Source: CAD feature listing. Evaluate the final solid. Frame: model axes, mm. Give positions to 0.01 mm unless a question says otherwise; leave off trailing zeros. Write each loop counter-clockwise with the first axis right and the second up, starting at its lowest first coordinate (ties: lowest second). Pieces come first, ordered by that corner, then holes. Notation, with made-up numbers: (-36.5, 14.25) -> (-17.5, 14.25) arc R5 ccw to (-17.5, 21.25) -> close; hole circle Ø3 at (18, -29.75). An arc over 180 degrees is marked (long way). Use one line per item in the form item = value. Start each with the question number.
(1) Cut plane A-A, the plane z = -390.5. Output: boundary loops of the cut face in (x, y) (3 decimals), and give its area (3 significant figures).
(2) Material intervals for line 1 along Z through (x, y) = (0.5, 4.25); line 2 along Z through (x, y) = (-2.25, -4.25); line 3 along Y through (x, z) = (-0.5, -454.5), sorted ascending. Write a range as from..to.
(3) First-contact query: P1, Ø6, axis at y = -1, z = -498.5, coming from the +X side; P2, Ø6, axis at x = -4.5, y = 4.5, coming from the -Z side; P3, Ø3, axis at x = 3, z = -450.5, coming from the -Y side. Flat tips, straight axial feed; report the tip coordinate or a pass-through.
from build123d import *

# Parameters (mm, degrees)
EXTRUDE1_DEPTH          = 7.9375
SKETCH13_R              = 6.35
EXTRUDE3_DEPTH          = 1.5875
SKETCH2_OUTSIDE_W       = 63.61
SKETCH2_OUTSIDE_H       = 63.61
SKETCH2_OUTSIDE_R       = 4.7625
CUT_EXTRUDE1_DEPTH      = 12.985362166
CUT_EXTRUDE1_DRAFT      = -60
SKETCH14_R              = 1.905
BOSS_EXTRUDE1_DEPTH     = 4.826
MIRROR1_COPY_1_SKETCH_W = 63.61
MIRROR1_COPY_1_SKETCH_H = 63.61
MIRROR1_COPY_1_SKETCH_R = 4.7625
MIRROR1_COPY_1_DEPTH    = 12.985362166
MIRROR1_COPY_1_DRAFT    = -60
SKETCH15_R              = 1.905
BOSS_EXTRUDE2_DEPTH     = 225.298
MIRROR2_COPY_1_SKETCH_W = 63.61
MIRROR2_COPY_1_SKETCH_H = 63.61
MIRROR2_COPY_1_SKETCH_R = 4.7625
MIRROR2_COPY_1_DEPTH    = 12.985362166
MIRROR2_COPY_1_DRAFT    = -60
MIRROR2_COPY_2_DEPTH    = 7.9375
MIRROR2_COPY_3_SKETCH_R = 6.35
MIRROR2_COPY_3_DEPTH    = 1.5875
MIRROR2_COPY_4_SKETCH_R = 1.905
MIRROR2_COPY_4_DEPTH    = 4.826
MIRROR2_COPY_5_SKETCH_W = 63.61
MIRROR2_COPY_5_SKETCH_H = 63.61
MIRROR2_COPY_5_SKETCH_R = 4.7625
MIRROR2_COPY_5_DEPTH    = 12.985362166
MIRROR2_COPY_5_DRAFT    = -60
SKETCH16_R              = 1.905
BOSS_EXTRUDE3_DEPTH     = 3.175
SKETCH4_R               = 1.905
BOSS_EXTRUDE4_DEPTH     = 3.175


with BuildPart() as part:
    # Sketch1 → Extrude1 (new body)
    with BuildSketch(Plane.XY):
        Polygon((0, 5.499261314), (-4.7625, 2.749630657), (-4.7625, -2.749630657), (0, -5.499261314), (4.7625, -2.749630657), (4.7625, 2.749630657), align=None)
    extrude1 = extrude(amount=-EXTRUDE1_DEPTH)

    # Sketch13 → Extrude3 (add)
    with BuildSketch(Plane(origin=(0, 0, -7.9375), x_dir=(-1, 0, 0), z_dir=(0, 0, -1))):
        Circle(SKETCH13_R)
    extrude3 = extrude(amount=-EXTRUDE3_DEPTH)


with BuildPart() as cut_extrude1_tool:
    # Sketch2 outside → Cut-Extrude1 (with draft: the straight prism first)
    with BuildSketch(Plane.XY):
        Rectangle(SKETCH2_OUTSIDE_W, SKETCH2_OUTSIDE_H)
        Circle(SKETCH2_OUTSIDE_R, mode=Mode.SUBTRACT)
    extrude(amount=-CUT_EXTRUDE1_DEPTH)
    # Cut-Extrude1: the draft: its side faces are tilted about the plane it starts from
    cut_extrude1_sides = [cut_extrude1_tool.faces().sort_by_distance(p)[0] for p in [
        (0, -31.805, -6.492681083),
        (31.805, 0, -6.492681083),
        (0, 31.805, -6.492681083),
        (-31.805, 0, -6.492681083),
        (-4.7625, 0, -6.492681083),
    ]]
    draft(cut_extrude1_sides, Plane.XY, CUT_EXTRUDE1_DRAFT)


with BuildPart() as part_1:
    add(part.part)

    # Cut-Extrude1: cut by cut_extrude1_tool
    add(cut_extrude1_tool.part, mode=Mode.SUBTRACT)

    # Sketch14 → Boss-Extrude1 (add)
    with BuildSketch(Plane(origin=(0, 0, -7.9375), x_dir=(-1, 0, 0), z_dir=(0, 0, -1))):
        Circle(SKETCH14_R)
    boss_extrude1 = extrude(amount=BOSS_EXTRUDE1_DEPTH)

    # Mirror1: Extrude1, Extrude3, Boss-Extrude1 across plane
    add(extrude1.mirror(Plane(origin=(0, 0, -12.7635), x_dir=(1, 0, 0), z_dir=(0, 0, -1))))
    add(extrude3.mirror(Plane(origin=(0, 0, -12.7635), x_dir=(1, 0, 0), z_dir=(0, 0, -1))))
    add(boss_extrude1.mirror(Plane(origin=(0, 0, -12.7635), x_dir=(1, 0, 0), z_dir=(0, 0, -1))))


with BuildPart() as mirror1_copy_1_tool:
    # Mirror1 copy 1 sketch → Mirror1 copy 1 (with draft: the straight prism first)
    with BuildSketch(Plane(origin=(0, 0, -25.527), x_dir=(1, 0, 0), z_dir=(0, 0, -1))):
        Rectangle(MIRROR1_COPY_1_SKETCH_W, MIRROR1_COPY_1_SKETCH_H)
        Circle(MIRROR1_COPY_1_SKETCH_R, mode=Mode.SUBTRACT)
    extrude(amount=-MIRROR1_COPY_1_DEPTH)
    # Mirror1 copy 1: the draft: its side faces are tilted about the plane it starts from
    mirror1_copy_1_sides = [mirror1_copy_1_tool.faces().sort_by_distance(p)[0] for p in [
        (0, -31.805, -19.034318917),
        (31.805, 0, -19.034318917),
        (0, 31.805, -19.034318917),
        (-31.805, 0, -19.034318917),
        (-4.7625, 0, -19.034318917),
    ]]
    draft(mirror1_copy_1_sides, Plane(origin=(0, 0, -25.527), x_dir=(1, 0, 0), z_dir=(0, 0, -1)), MIRROR1_COPY_1_DRAFT)


with BuildPart() as part_2:
    add(part_1.part)

    # Mirror1 copy 1: cut by mirror1_copy_1_tool
    add(mirror1_copy_1_tool.part, mode=Mode.SUBTRACT)

    # Sketch15 → Boss-Extrude2 (add)
    with BuildSketch(Plane(origin=(0, 0, -25.527), x_dir=(-1, 0, 0), z_dir=(0, 0, -1))):
        Circle(SKETCH15_R)
    boss_extrude2 = extrude(amount=BOSS_EXTRUDE2_DEPTH)

    # Mirror2: Extrude1, Extrude3, Boss-Extrude1, Boss-Extrude2 across plane
    add(extrude1.mirror(Plane(origin=(0, 0, -250.825), x_dir=(1, 0, 0), z_dir=(0, 0, -1))))
    add(extrude3.mirror(Plane(origin=(0, 0, -250.825), x_dir=(1, 0, 0), z_dir=(0, 0, -1))))
    add(boss_extrude1.mirror(Plane(origin=(0, 0, -250.825), x_dir=(1, 0, 0), z_dir=(0, 0, -1))))
    add(boss_extrude2.mirror(Plane(origin=(0, 0, -250.825), x_dir=(1, 0, 0), z_dir=(0, 0, -1))))


with BuildPart() as mirror2_copy_1_tool:
    # Mirror2 copy 1 sketch → Mirror2 copy 1 (with draft: the straight prism first)
    with BuildSketch(Plane(origin=(0, 0, -501.65), x_dir=(1, 0, 0), z_dir=(0, 0, -1))):
        Rectangle(MIRROR2_COPY_1_SKETCH_W, MIRROR2_COPY_1_SKETCH_H)
        Circle(MIRROR2_COPY_1_SKETCH_R, mode=Mode.SUBTRACT)
    extrude(amount=-MIRROR2_COPY_1_DEPTH)
    # Mirror2 copy 1: the draft: its side faces are tilted about the plane it starts from
    mirror2_copy_1_sides = [mirror2_copy_1_tool.faces().sort_by_distance(p)[0] for p in [
        (0, -31.805, -495.157318917),
        (31.805, 0, -495.157318917),
        (0, 31.805, -495.157318917),
        (-31.805, 0, -495.157318917),
        (-4.7625, 0, -495.157318917),
    ]]
    draft(mirror2_copy_1_sides, Plane(origin=(0, 0, -501.65), x_dir=(1, 0, 0), z_dir=(0, 0, -1)), MIRROR2_COPY_1_DRAFT)


with BuildPart() as part_3:
    add(part_2.part)

    # Mirror2 copy 1: cut by mirror2_copy_1_tool
    add(mirror2_copy_1_tool.part, mode=Mode.SUBTRACT)

    # Mirror2 copy 2 sketch → Mirror2 copy 2 (add)
    with BuildSketch(Plane.XY.offset(-476.123)):
        Polygon((0, 5.499261314), (-4.7625, 2.749630657), (-4.7625, -2.749630657), (0, -5.499261314), (4.7625, -2.749630657), (4.7625, 2.749630657), align=None)
    extrude(amount=-MIRROR2_COPY_2_DEPTH)

    # Mirror2 copy 3 sketch → Mirror2 copy 3 (add)
    with BuildSketch(Plane(origin=(0, 0, -484.0605), x_dir=(-1, 0, 0), z_dir=(0, 0, -1))):
        Circle(MIRROR2_COPY_3_SKETCH_R)
    extrude(amount=-MIRROR2_COPY_3_DEPTH)

    # Mirror2 copy 4 sketch → Mirror2 copy 4 (add)
    with BuildSketch(Plane(origin=(0, 0, -484.0605), x_dir=(-1, 0, 0), z_dir=(0, 0, -1))):
        Circle(MIRROR2_COPY_4_SKETCH_R)
    extrude(amount=MIRROR2_COPY_4_DEPTH)


with BuildPart() as mirror2_copy_5_tool:
    # Mirror2 copy 5 sketch → Mirror2 copy 5 (with draft: the straight prism first)
    with BuildSketch(Plane.XY.offset(-476.123)):
        Rectangle(MIRROR2_COPY_5_SKETCH_W, MIRROR2_COPY_5_SKETCH_H)
        Circle(MIRROR2_COPY_5_SKETCH_R, mode=Mode.SUBTRACT)
    extrude(amount=-MIRROR2_COPY_5_DEPTH)
    # Mirror2 copy 5: the draft: its side faces are tilted about the plane it starts from
    mirror2_copy_5_sides = [mirror2_copy_5_tool.faces().sort_by_distance(p)[0] for p in [
        (0, -31.805, -482.615681083),
        (31.805, 0, -482.615681083),
        (0, 31.805, -482.615681083),
        (-31.805, 0, -482.615681083),
        (-4.7625, 0, -482.615681083),
    ]]
    draft(mirror2_copy_5_sides, Plane.XY.offset(-476.123), MIRROR2_COPY_5_DRAFT)


with BuildPart() as part_4:
    add(part_3.part)

    # Mirror2 copy 5: cut by mirror2_copy_5_tool
    add(mirror2_copy_5_tool.part, mode=Mode.SUBTRACT)

    # Sketch16 → Boss-Extrude3 (add)
    with BuildSketch(Plane(origin=(0, 0, -501.65), x_dir=(-1, 0, 0), z_dir=(0, 0, -1))):
        Circle(SKETCH16_R)
    extrude(amount=BOSS_EXTRUDE3_DEPTH)

    # Sketch4 → Boss-Extrude4 (add)
    with BuildSketch(Plane.XY):
        with Locations(Location((0, 0, 0), (0, 0, 180))):
            Circle(SKETCH4_R)
    extrude(amount=BOSS_EXTRUDE4_DEPTH)


solid = part_4.part
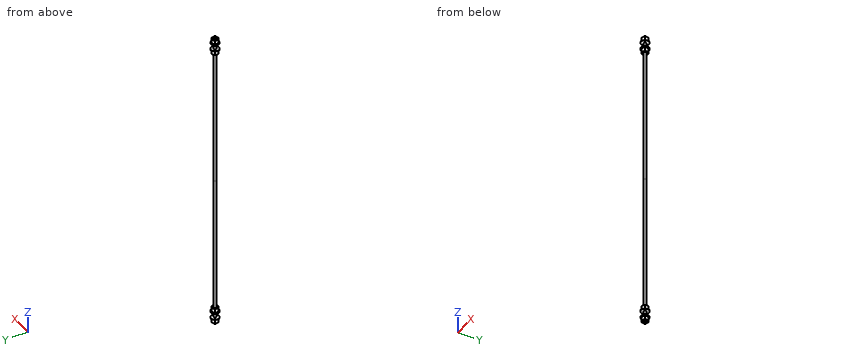
Geometry says:
q1.outline = circle Ø3.81 at (0, 0)
q1.area = 11.4 mm^2
q2.line_1 = -501.65..-493.71, -484.06..-476.12, -25.53..-17.59, -7.94..0
q2.line_2 = -495.3..-493.71, -484.06..-482.47, -19.18..-17.59, -7.94..-6.35
q2.line_3 = -1.84..1.84
q3.P1 = 4.76
q3.P2 = -501.65
q3.P3 = -1.17
